```python
from build123d import *

# Parameters (mm, degrees)
SKETCH1_W           = 26.67
SKETCH1_H           = 20.32
SKETCH1_R           = 1.707818092
SKETCH1_R_2         = 1.06997981
BOSS_EXTRUDE1_DEPTH = 1.6
SKETCH2_W           = 9.449727346
SKETCH2_H           = 9.64726846
BOSS_EXTRUDE2_DEPTH = 1.6


with BuildPart() as part:
    # Sketch1 → Boss-Extrude1 (new body)
    with BuildSketch(Plane(origin=(0, 0, 0), x_dir=(1, 0, 0), z_dir=(0, 1, 0))):
        Rectangle(SKETCH1_W, SKETCH1_H)
        with Locations(Location((-10.795, 7.62, 0), (0, 0, 270))):
            Circle(SKETCH1_R, mode=Mode.SUBTRACT)
        with Locations(Location((10.795, 7.62, 0), (0, 0, 90))):
            Circle(SKETCH1_R, mode=Mode.SUBTRACT)
        with Locations(Location((10.795, -7.62, 0), (0, 0, 270))):
            Circle(SKETCH1_R, mode=Mode.SUBTRACT)
        with Locations(Location((-10.795, -7.62, 0), (0, 0, 90))):
            Circle(SKETCH1_R, mode=Mode.SUBTRACT)
        with Locations(Location((-1.27, -7.62, 0), (0, 0, 270))):
            Circle(SKETCH1_R_2, mode=Mode.SUBTRACT)
        with Locations(Location((-3.81, -7.62, 0), (0, 0, 270))):
            Circle(SKETCH1_R_2, mode=Mode.SUBTRACT)
        with Locations(Location((-6.35, -7.62, 0), (0, 0, 270))):
            Circle(SKETCH1_R_2, mode=Mode.SUBTRACT)
        with Locations(Location((6.35, -7.62, 0), (0, 0, 90))):
            Circle(SKETCH1_R_2, mode=Mode.SUBTRACT)
        with Locations(Location((3.81, -7.62, 0), (0, 0, 90))):
            Circle(SKETCH1_R_2, mode=Mode.SUBTRACT)
        with Locations(Location((1.27, -7.62, 0), (0, 0, 90))):
            Circle(SKETCH1_R_2, mode=Mode.SUBTRACT)
    extrude(amount=BOSS_EXTRUDE1_DEPTH)

    # Sketch2 → Boss-Extrude2 (add)
    with BuildSketch(Plane(origin=(0, 1.6, 0), x_dir=(1, 0, 0), z_dir=(0, 1, 0))):
        Rectangle(SKETCH2_W, SKETCH2_H)
    extrude(amount=BOSS_EXTRUDE2_DEPTH)


solid = part.part
```
CAD build for the part. Positions are in the model's coordinates, mm. A direction names the side the tool comes from. Coordinates: 2 decimals unless noted, no trailing zeros. Loops run counter-clockwise (first coordinate to the right, second up) from the corner with the lowest first, then second, coordinate; pieces in that order, holes last. Notation, with made-up numbers: (88.25, -36) - (133.25, -36) arc R14 ccw to (133.25, -15) - close; hole circle Ø3 at (4.5, 35.25). An arc over 180 degrees is marked (long way). Return JSON: item names as keys, results as strings.
1. Drop flat-ended pins along their axis: pin 1 (1.5 mm diameter, centred on x = -6, z = -4, fed in from +Y); pin 2 (12 mm diameter, centred on x = 9, z = -8, fed in from -Y); pin 3 (1.3 mm diameter, centred on x = -2, y = 3, fed in from -Z); pin 4 (1.3 mm diameter, centred on x = -1, y = 3, fed in from +Z). Give the stop position or say it passes through.
Result:
{"pin 1": "stops at y = 1.6", "pin 2": "stops at y = 0", "pin 3": "stops at z = -4.82", "pin 4": "stops at z = 4.82"}
2. Band-saw the part on A-A (z = -7.62). Give the cut face in (x, y) (3 decimals).
Result:
{"outline": "(-13.335, 0) - (-12.503, 0) - (-12.503, 1.6) - (-13.335, 1.6) - close; (-9.087, 0) - (9.087, 0) - (9.087, 1.6) - (-9.087, 1.6) - close; (12.503, 0) - (13.335, 0) - (13.335, 1.6) - (12.503, 1.6) - close"}
3. Band-saw the part on B-B (x = -3.81). Give the cut face in (y, z).
Result:
{"outline": "(0, -10.16) - (1.6, -10.16) - (1.6, -4.82) - (3.2, -4.82) - (3.2, 4.82) - (1.6, 4.82) - (1.6, 6.55) - (0, 6.55) - close; (0, 8.69) - (1.6, 8.69) - (1.6, 10.16) - (0, 10.16) - close"}
4. 3-axis set-ups, long thin cutter, end or side, ignore diameter. For faces 1 (the flat face through (0, 1, 10.16)), 2 (the flat face through (4.725, 2, 0)), 3 (the flat face through (0, 2, 4.824)), 4 (the flat face through (-4.725, 2, 0)): which of +Z, -Z, +X, -X, +Y, -Y reach the whole face in a straight line?
Result:
{"face 1": "+Z, +X, -X, +Y, -Y", "face 2": "+Z, -Z, +X, +Y", "face 3": "+Z, +X, -X, +Y", "face 4": "+Z, -Z, -X, +Y"}
5. Probe L1, parallel to X at y = 2.65, z = -4.75; L2, parallel to Y at x = -5.75, z = -6.75; L3, parallel to X at y = 1.4, z = -8.75 (3 decimals). List the from-to ranges inside material, lowest first. Write a range as from..to.
Result:
{"L1": "x = -4.72..4.72", "L2": "y = 0..1.6", "L3": "x = -13.335..-12.076, -9.514..9.514, 12.076..13.335"}
6. Band-saw the part on D-D (x = 6.35). Give the cut face in (y, z).
Result:
{"outline": "(0, -10.16) - (1.6, -10.16) - (1.6, 6.55) - (0, 6.55) - close; (0, 8.69) - (1.6, 8.69) - (1.6, 10.16) - (0, 10.16) - close"}
7. Mould opens along Z. For faces 5 (the flat face through (-13.335, 1, 0)), 6 (the cylindrical face through (9.28, 0.79, 8.41)), 7 (the flat face through (0, 2, -4.824)) say: released by +Z, released by -Z, zero draft, split by the parting line, or undercut.
Result:
{"face 5": "zero draft", "face 6": "undercut", "face 7": "released by -Z"}
8. Band-saw the part on C-C (z = 4). Give the cut face in (x, y) (3 decimals).
Result:
{"outline": "(-13.335, 0) - (13.335, 0) - (13.335, 1.6) - (4.725, 1.6) - (4.725, 3.2) - (-4.725, 3.2) - (-4.725, 1.6) - (-13.335, 1.6) - close"}
